Geometry check sheet. Reference: the model listing, model coordinates, mm. Face numbers are marked on the shaded views. A direction names the side the tool comes from. Round coordinates to 2 decimals unless told otherwise and drop trailing zeros. Order: outer loops, then holes, each group sorted by start corner. A loop starts at its lowest first (then second) coordinate and runs counter-clockwise, first axis right, second up.
(1) Cross-section at D-D on y = 117.5. Enter the section's corners in (x, z).
(2) Draft check along Y on the marked faces 3 and 4. Enter one of: pulls with the +Y half, pulls with the -Y half, needs draft (parallel to the pull), parting line crosses it, or undercut.
(3) Cross-section at A-A on y = 208.5. Enter the section's corners in (x, z), and give its area (3 significant figures).
(4) Set-up check for the marked faces 1 and 2: record each of +Z, -Z, +X, -X, +Y, -Y from which the full face is reachable in a straight line by a thin tool's end or side.
(5) Thickness scan on L1, parallel to X at y = 144, z = 5.5; L2, parallel to X at y = 216, z = 3.25; L3, parallel to Z at x = -59, y = 42. Record the ranges inside material, lowest first.
(6) Cross-section at B-B on x = -217.5. Enter the section's corners in (y, z).
(7) Gauge pin test, flat ends, axial feed: P1, Ø6, axis at x = -179, y = 143, coming from the +Z side; P2, Ø0.8, axis at y = 199, z = 0.5, coming from the +X side; P3, Ø10, axis at x = -67, y = 54, coming from the -Z side. Record the tip position at first contact, or that the pin passes through.
(8) Cross-section at C-C on y = 35. Enter the section's corners in (x, z), and give its area (3 significant figures).
from build123d import *
from build123d import SkipClean  # not in build123d's __all__

# Parameters (mm, degrees)
F0_R     = 10
F1_DEPTH = 10
F2_DEPTH = 1
F4_DEPTH = 345
F5_DEPTH = 7.3
F6_DEPTH = 1.6


with BuildPart() as f1:
    # F0 (on Top) → F1 (new body)
    with BuildSketch(Plane.XY):
        Polygon((-255.5560874402, 235.83927431), (-264.2086340252, 225.0363213116), (-264.2086340252, 185.7455475346), (-236.384913462, 220.4842620314), align=None)
        Polygon((-264.2086340252, 185.7455475346), (-264.2086340252, 225.0363213116), (-283.3798080034, 201.1005598132), align=None)
        Polygon((-236.384913462, 220.4842620314), (-264.2086340252, 185.7455475346), (-236.8907927142, 163.8655213438), (-209.0670721511, 198.6042358405), align=None)
        Polygon((-209.0670721511, 198.6042358405), (-236.8907927142, 163.8655213438), (-108.6030207612, 61.1143640196), (-80.779300198, 95.8530785163), align=None)
        with Locations((-175.4610245732, 143.8843668861)):
            Circle(F0_R, mode=Mode.SUBTRACT)
        with Locations((-118.6635494232, 98.6492335796)):
            Circle(F0_R, mode=Mode.SUBTRACT)
        Polygon((-80.779300198, 95.8530785163), (-108.6030207612, 61.1143640196), (-52.4192279143, 16.1143640196), (-31.023575784, 16.1143640196), (-24.2086340252, 24.6230145983), (-24.2086340252, 50.5432151414), align=None)
        Polygon((-11.5613729408, 40.4134834171), (-24.2086340252, 50.5432151414), (-24.2086340252, 24.6230145983), align=None)
        Polygon((-31.023575784, 16.1143640196), (-52.4192279143, 16.1143640196), (-39.385093504, 5.6747689203), align=None)
    extrude(amount=F1_DEPTH)

    # F0 (on Top) → F2 (cut)
    with BuildSketch(Plane.XY):
        Polygon((-255.5560874402, 235.83927431), (-264.2086340252, 225.0363213116), (-264.2086340252, 185.7455475346), (-236.384913462, 220.4842620314), align=None)
        Polygon((-236.384913462, 220.4842620314), (-264.2086340252, 185.7455475346), (-236.8907927142, 163.8655213438), (-209.0670721511, 198.6042358405), align=None)
        Polygon((-209.0670721511, 198.6042358405), (-236.8907927142, 163.8655213438), (-108.6030207612, 61.1143640196), (-80.779300198, 95.8530785163), align=None)
        with Locations((-175.4610245732, 143.8843668861)):
            Circle(F0_R, mode=Mode.SUBTRACT)
        with Locations((-118.6635494232, 98.6492335796)):
            Circle(F0_R, mode=Mode.SUBTRACT)
        Polygon((-80.779300198, 95.8530785163), (-108.6030207612, 61.1143640196), (-52.4192279143, 16.1143640196), (-31.023575784, 16.1143640196), (-24.2086340252, 24.6230145983), (-24.2086340252, 50.5432151414), align=None)
    extrude(amount=F2_DEPTH, mode=Mode.SUBTRACT)

    # F3 (on face) → F4 (cut)
    with BuildSketch(Plane(origin=(-270.7568290083, 216.860711746, 0), x_dir=(-0.6251436055, -0.7805097517, 0), z_dir=(-0.7805097517, 0.6251436055, 0))):
        Polygon((20.192126873, 10), (-24.3155995446, 10), (20.192126873, 0), align=None)
        Polygon((-17.6889132261, 39.4938741719), (-24.3155995446, 10), (20.192126873, 10), (20.192126873, 0), (26.8188131915, 29.4938741719), align=None)
    extrude(amount=-F4_DEPTH, mode=Mode.SUBTRACT)

    # F0 (on Top) → F5 (join)
    with BuildSketch(Plane.XY):
        with Locations((-175.4610245732, 143.8843668861)):
            Circle(F0_R)
        with Locations((-118.6635494232, 98.6492335796)):
            Circle(F0_R)
    with SkipClean():  # cleaning this boolean's faces spoils the solid; the shape is the same uncleaned
        extrude(amount=F5_DEPTH)

    # F0 (on Top) → F6 (cut)
    with BuildSketch(Plane.XY):
        with Locations((-118.6635494232, 98.6492335796)):
            Circle(F0_R)
        with Locations((-175.4610245732, 143.8843668861)):
            Circle(F0_R)
    with SkipClean():  # cleaning this boolean's faces spoils the solid; the shape is the same uncleaned
        extrude(amount=F6_DEPTH, mode=Mode.SUBTRACT)


solid = f1.part
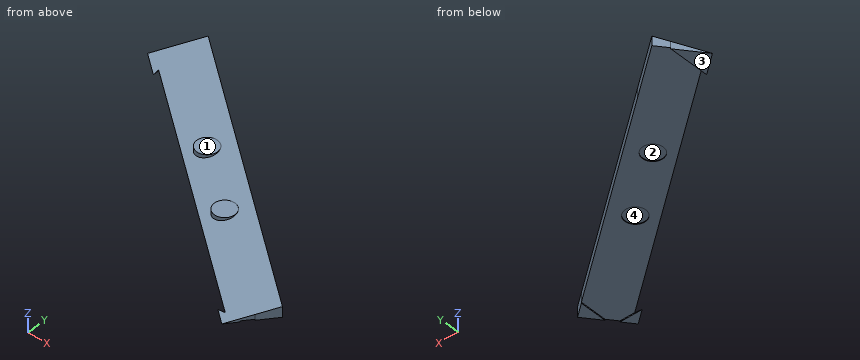
Found:
1. outline: (-171.88, 1) - (-107.81, 1) - (-107.81, 10) - close
2. face 3: needs draft
2. face 4: undercut
3. outline: (-277.45, 0) - (-264.21, 0) - (-264.21, 1) - (-221.42, 1) - (-221.42, 10) - (-277.45, 2.13) - close
3. area: 297 mm2
4. face 1: +Z, -X, -Y
4. face 2: -Z
5. L1: x = -185.46 to -140.89
5. L2: x = -271.45 to -230.79
5. L3: z = 1 to 3.62
6. outline: (154.04, 1) - (205.36, 1) - (205.36, 10) - close
7. P1: stops at z = 7.3
7. P2: stops at x = -264.21
7. P3: stops at z = 1
8. outline: (-68.88, 1) - (-24.21, 1) - (-24.21, 0) - (-15.9, 0) - (-15.9, 8.44) - close
8. area: 205 mm2
